from build123d import *

# Parameters (mm, degrees)
SKETCH1_W           = 50
SKETCH1_H           = 43
SKETCH1_R           = 2.75
BOSS_EXTRUDE1_DEPTH = 6
SKETCH2_R           = 7
CUT_EXTRUDE1_DEPTH  = 6
SKETCH3_R           = 2.25
CUT_EXTRUDE2_DEPTH  = 6
SKETCH4_R           = 12.75
CUT_EXTRUDE3_DEPTH  = 3
FILLET1_R           = 5


with BuildPart() as part:
    # Sketch1 → Boss-Extrude1 (new body)
    with BuildSketch(Plane(origin=(0, 0, 0), x_dir=(1, 0, 0), z_dir=(0, 1, 0))):
        Rectangle(SKETCH1_W, SKETCH1_H)
        with Locations(Location((-20, 16.5, 0), (0, 0, 270))):
            Circle(SKETCH1_R, mode=Mode.SUBTRACT)
        with Locations(Location((20, 16.5, 0), (0, 0, 270))):
            Circle(SKETCH1_R, mode=Mode.SUBTRACT)
        with Locations(Location((-20, -16.5, 0), (0, 0, 270))):
            Circle(SKETCH1_R, mode=Mode.SUBTRACT)
        with Locations(Location((20, -16.5, 0), (0, 0, 270))):
            Circle(SKETCH1_R, mode=Mode.SUBTRACT)
    extrude(amount=BOSS_EXTRUDE1_DEPTH)

    # Sketch2 → Cut-Extrude1 (cut)
    with BuildSketch(Plane(origin=(0, 6, 0), x_dir=(1, 0, 0), z_dir=(0, 1, 0))):
        with Locations(Location((0, 0, 0), (0, 0, 270))):
            Circle(SKETCH2_R)
    extrude(amount=-CUT_EXTRUDE1_DEPTH, mode=Mode.SUBTRACT)

    # Sketch3 → Cut-Extrude2 (cut)
    with BuildSketch(Plane(origin=(0, 6, 0), x_dir=(1, 0, 0), z_dir=(0, 1, 0))):
        with Locations(Location((0, 17.5, 0), (0, 0, 270))):
            Circle(SKETCH3_R)
        with Locations(Location((17.5, 0, 0), (0, 0, 270))):
            Circle(SKETCH3_R)
        with Locations(Location((0, -17.5, 0), (0, 0, 270))):
            Circle(SKETCH3_R)
        with Locations(Location((-17.5, 0, 0), (0, 0, 270))):
            Circle(SKETCH3_R)
    extrude(amount=-CUT_EXTRUDE2_DEPTH, mode=Mode.SUBTRACT)

    # Sketch4 → Cut-Extrude3 (cut)
    with BuildSketch(Plane(origin=(0, 6, 0), x_dir=(1, 0, 0), z_dir=(0, 1, 0))):
        with Locations(Location((0, 0, 0), (0, 0, 270))):
            Circle(SKETCH4_R)
    extrude(amount=-CUT_EXTRUDE3_DEPTH, mode=Mode.SUBTRACT)

    # Fillet1
    fillet1_edges = [part.edges().sort_by_distance(p)[0] for p in [
        (-25, 3, -21.5),
        (25, 3, -21.5),
        (25, 3, 21.5),
        (-25, 3, 21.5),
    ]]
    fillet(fillet1_edges, radius=FILLET1_R)


solid = part.part
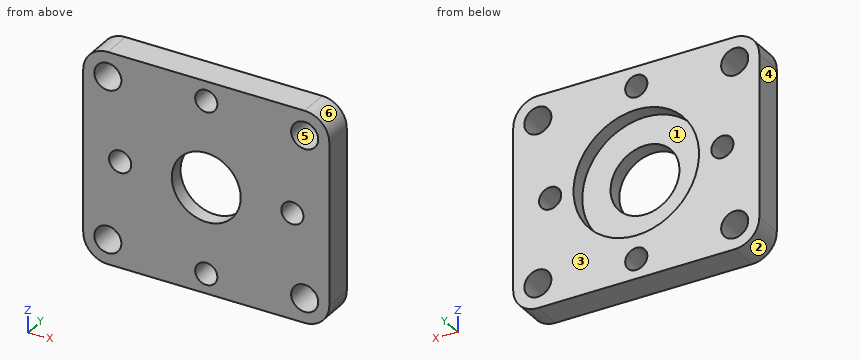
Input: part model. Units: mm. Frame: model coordinates. Face numbers are marked on the shaded views. A direction names the side the tool comes from. Round coordinates to 2 decimals unless told otherwise and drop trailing zeros. Write each loop counter-clockwise with the first axis right and the second up, starting at its lowest first coordinate (ties: lowest second). Pieces come first, ordered by that corner, then holes.
1) Ray query, L1, parallel to X at y = 2.4, z = 0; L2, parallel to X at y = 1.25, z = -17.5; L3, parallel to X at y = 5.35, z = -15. Return the intervals inside material, ascending.
2) Cut plane D-D (x = -5.5). Return the cut outline in (y, z).
3) Cut plane C-C (y = 1.95). Count the separate pieces of the cut face and the enclosed holes in it, then the cut area to 3 significant figures.
4) Reachability of the marked faces 1 and 2 from +Z, -Z, +X, -X, +Y, -Y: full face, straight path, thin tool, end or side. Return the list, or none.
5) Contact query for flat-ended pins moving along their axis: P1, Ø12.5, axis at x = 0, z = 0, coming from the +Y side; P2, Ø1, axis at x = 6, z = -3, coming from the +Y side. Output: stop coordinate, or through.
6) Draft query along X for the marked faces 3, 4, 5 and 6. Return one class per face: pulls with the +X half, pulls with the -X half, needs draft (parallel to the pull), parting line crosses it, or undercut.
7) Cut plane B-B (x = 0). Return the cut outline in (y, z).
8) Cut plane A-A (z = 0). Return the cut outline in (x, y), then the cut area to 4 significant figures.
Geometry says:
1. L1: x = -25 to -19.75, -15.25 to -7, 7 to 15.25, 19.75 to 25
1. L2: x = -24.9 to -22.56, -17.44 to -2.25, 2.25 to 17.44, 22.56 to 24.9
1. L3: x = -25 to -22.3, -17.7 to 17.7, 22.3 to 25
2. outline: (0, -21.5) - (6, -21.5) - (6, -11.5) - (3, -11.5) - (3, -4.33) - (0, -4.33) - close; (0, 4.33) - (3, 4.33) - (3, 11.5) - (6, 11.5) - (6, 21.5) - (0, 21.5) - close
3. separate pieces: 1
3. enclosed holes: 9
3. area: 1,820 mm2
4. face 1: +Y
4. face 2: -Z, -X, +Y, -Y
5. P1: passes through
5. P2: stops at y = 3
6. face 3: needs draft
6. face 4: pulls with the -X half
6. face 5: undercut
6. face 6: pulls with the +X half
7. outline: (0, -21.5) - (6, -21.5) - (6, -19.75) - (0, -19.75) - close; (0, -15.25) - (6, -15.25) - (6, -12.75) - (3, -12.75) - (3, -7) - (0, -7) - close; (0, 7) - (3, 7) - (3, 12.75) - (6, 12.75) - (6, 15.25) - (0, 15.25) - close; (0, 19.75) - (6, 19.75) - (6, 21.5) - (0, 21.5) - close
8. outline: (-25, 0) - (-19.75, 0) - (-19.75, 6) - (-25, 6) - close; (-15.25, 0) - (-7, 0) - (-7, 3) - (-12.75, 3) - (-12.75, 6) - (-15.25, 6) - close; (7, 0) - (15.25, 0) - (15.25, 6) - (12.75, 6) - (12.75, 3) - (7, 3) - close; (19.75, 0) - (25, 0) - (25, 6) - (19.75, 6) - close
8. area: 127.5 mm2
